```python
from build123d import *

# Parameters (mm, degrees)
F0_R     = 6.35
F1_DEPTH = 50
F2_DEPTH = 55
F3_R     = 3
F4_DEPTH = 10


with BuildPart() as f1:
    # F0 (on Top) → F1 (new body, symmetric)
    with BuildSketch(Plane.XY):
        with BuildLine():
            ThreePointArc((10, -14.361407), (15.512092, -8.100926), (17.5, 0))
            ThreePointArc((17.5, 0), (-8.100926, 15.512092), (-10, -14.361407))
            Line((-10, -14.361407), (10, -14.361407))
        make_face()
        Circle(F0_R, mode=Mode.SUBTRACT)
        Circle(F0_R)
    extrude(amount=F1_DEPTH, both=True)

    # F0 (on Top) → F2 (join, symmetric)
    with BuildSketch(Plane.XY):
        Circle(F0_R)
    extrude(amount=F2_DEPTH, both=True)

    # F3 (on face) → F4 (cut)
    with BuildSketch(Plane.XZ.offset(14.361407)):
        with Locations((0, 21)):
            Circle(F3_R)
        with Locations((0, -21)):
            Circle(F3_R)
    extrude(amount=-F4_DEPTH, mode=Mode.SUBTRACT)


solid = f1.part
```
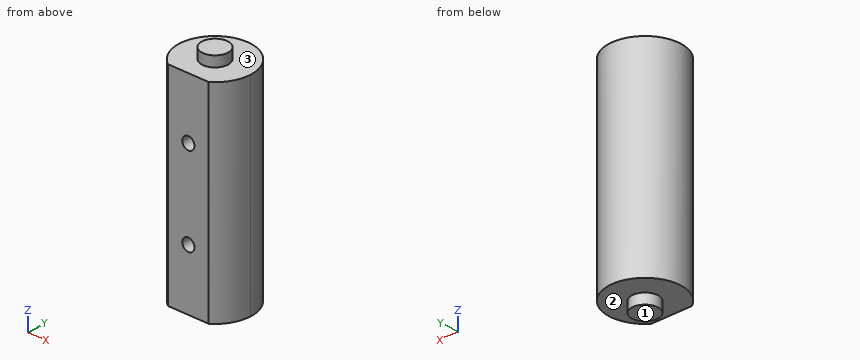
Verification items for the finished model (mm, model axes). Face numbers are marked on the shaded views. A direction names the side the tool comes from. Round coordinates to 2 decimals unless told otherwise and drop trailing zeros. Order: outer loops, then holes, each group sorted by start corner. A loop starts at its lowest first (then second) coordinate and runs counter-clockwise, first axis right, second up.
1) Cross-section at A-A, the plane z = 21. Record the cut outline in (x, y), plus the area to 3 significant figures.
Geometry says:
outline: (-10, -14.36) - (-3, -14.36) - (-3, -4.36) - (3, -4.36) - (3, -14.36) - (10, -14.36) arc R17.5 ccw to (17.5, 0) arc R17.5 ccw (long way) to start
area: 859 mm2
2) Material ranges on line 1 (Z direction, x = 0, y = -9); line 2 (Z direction, x = -2.5, y = 12); line 3 (Y direction, x = -8, z = -37.5), recorded low to high.
Geometry says:
line 1: z = -50 to -24, -18 to 18, 24 to 50
line 2: z = -50 to 50
line 3: y = -14.36 to 15.56
3) Cross-section at D-D, the plane y = -8. Record the cut outline in (x, z), plus the area to 3 significant figures.
Geometry says:
outline: (-15.56, -50) - (15.56, -50) - (15.56, 50) - (-15.56, 50) - close; hole circle Ø6 at (0, -21); hole circle Ø6 at (0, 21)
area: 3,060 mm2
4) Tool access check on the marked faces 1, 2 and 3. Record the directions out of +Z, -Z, +X, -X, +Y, -Y that give a thin tool (end or side, any length) a straight path to the whole face; none if there is none.
Geometry says:
face 1: -Z, +X, -X, +Y, -Y
face 2: -Z
face 3: +Z
5) Cross-section at B-B, the plane x = 0. Record the cut outline in (y, z).
Geometry says:
outline: (-14.36, -50) - (-6.35, -50) - (-6.35, -55) - (6.35, -55) - (6.35, -50) - (17.5, -50) - (17.5, 50) - (6.35, 50) - (6.35, 55) - (-6.35, 55) - (-6.35, 50) - (-14.36, 50) - (-14.36, 24) - (-4.36, 24) - (-4.36, 18) - (-14.36, 18) - (-14.36, -18) - (-4.36, -18) - (-4.36, -24) - (-14.36, -24) - close
6) Depth check by flat-ended pin: pin 1 (12 mm diameter, centred on x = 13, y = -2, fed in from -Z); pin 2 (5.5 mm diameter, centred on x = 0, z = -21, fed in from -Y); pin 3 (10 mm diameter, centred on x = -11.5, y = -0.5, fed in from +Z). Enter the tip coordinate at first touch or a pass-through.
Geometry says:
pin 1: stops at z = -50
pin 2: stops at y = -4.36
pin 3: stops at z = 50
7) Cross-section at C-C, the plane y = 2. Record the cut outline in (x, z).
Geometry says:
outline: (-17.39, -50) - (-6.03, -50) - (-6.03, -55) - (6.03, -55) - (6.03, -50) - (17.39, -50) - (17.39, 50) - (6.03, 50) - (6.03, 55) - (-6.03, 55) - (-6.03, 50) - (-17.39, 50) - close
